from build123d import *


with BuildPart() as part:
    # Sweep1: sweep along a path in Sketch4
    with BuildLine(Plane(origin=(0, 0, 0), x_dir=(0, 0, -1), z_dir=(1, 0, 0))) as sweep1_path:
        Line((0, 0), (-2.286, 6.35))
    # Sketch2 → Sweep1 (sweep)
    with BuildSketch(Plane(origin=(0, 0, 0), x_dir=(1, 0, 0), z_dir=(0, 1, 0))):
        with BuildLine():
            Line((6.9596, -10.377746103), (4.0132, -10.377746103))
            Line((4.0132, -10.377746103), (4.0132, -5.373946103))
            Line((4.0132, -5.373946103), (2.413, -5.373946103))
            Line((2.413, -5.373946103), (3.556, -3.773746103))
            Line((3.556, -3.773746103), (-3.556, -3.773746103))
            Line((-3.556, -3.773746103), (-2.413, -5.373946103))
            Line((-2.413, -5.373946103), (-4.0132, -5.373946103))
            Line((-4.0132, -5.373946103), (-4.0132, -10.377746103))
            Line((-4.0132, -10.377746103), (-6.9596, -10.377746103))
            ThreePointArc((-6.9596, -10.377746103), (-5.806615649, -2.567356115), (-5.877729648, 5.327357779))
            ThreePointArc((-5.877729648, 5.327357779), (-5.125150102, 6.465638091), (-3.98686979, 5.713058545))
            ThreePointArc((-3.98686979, 5.713058545), (-2.834757288, 3.806705335), (-0.7366, 3.058853897))
            Line((-0.7366, 3.058853897), (-0.7366, 1.407853897))
            Line((-0.7366, 1.407853897), (0.7366, 1.407853897))
            Line((0.7366, 1.407853897), (0.7366, 3.058853897))
            ThreePointArc((0.7366, 3.058853897), (2.834757288, 3.806705335), (3.98686979, 5.713058545))
            ThreePointArc((3.98686979, 5.713058545), (5.125150102, 6.465638091), (5.877729648, 5.327357779))
            ThreePointArc((5.877729648, 5.327357779), (5.806615649, -2.567356115), (6.9596, -10.377746103))
        make_face()
    sweep(path=sweep1_path.line)


solid = part.part
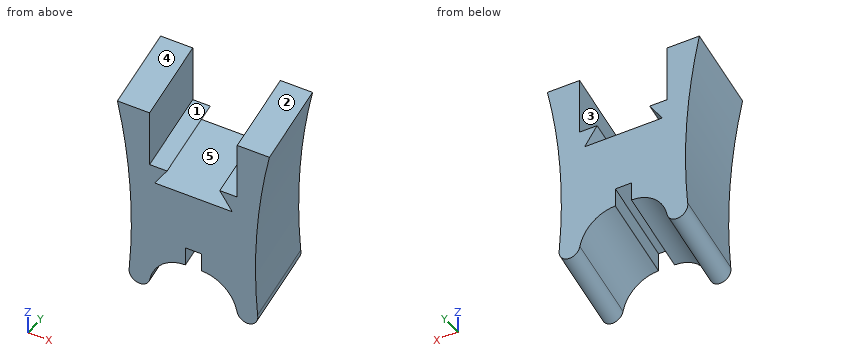
Read the model definition and answer for the solid it produces. Units are mm, in the model's axes. Face numbers are marked on the shaded views. A direction names the side the tool comes from. Round coordinates to 2 decimals unless told otherwise and drop trailing zeros. Write each loop counter-clockwise with the first axis right and the second up, starting at its lowest first coordinate (ties: lowest second). Pieces come first, ordered by that corner, then holes.
1. The part is cut by section A-A, the plane x = -0.5. Determine the outline of the cut face in (y, z), then the cut area to 3 significant figures.
2. Straight lines are drawn through the part: L1, parallel to X at y = 1.25, z = -3; L2, parallel to Z at x = -3, y = 2.5; L3, parallel to X at y = 1, z = -4.25. For each, find the intervals that lie inside material, in ascending order.
3. Given pin 1 Ø1.2 at (y, z) = (4.5, 0) entering from -X; pin 2 Ø4 at (x, z) = (-2.5, 8) entering from +Y; pin 3 Ø1.2 at (y, z) = (2.5, -0.5) entering from +X; pin 4 Ø3 at (x, y) = (5, 2.5) entering from -Z, each flat-ended and moving along its own axis, determine where each tip first touches the part or whether it passes through.
4. Determine the mould class of the marked faces 3, 4 and 5 for opening direction Z: pulls with the +Z half, pulls with the -Z half, needs draft (parallel to the pull), parting line crosses it, or undercut.
5. Which of the six approach directions +Z, -Z, +X, -X, +Y, -Y give full straight-line access (tool end or side, diameter ignored) to the marked faces 1 and 2?
Values:
1. outline: (0, -1.41) - (6.35, 0.88) - (6.35, 6.06) - (0, 3.77) - close
1. area: 32.9 mm2
2. L1: x = -5.75 to -2.3, 2.3 to 5.75
2. L2: z = -3.05 to 4.67, 5.45 to 6.27
2. L3: x = -5.82 to -3.54, 3.54 to 5.82
3. pin 1: stops at x = -5.7
3. pin 2: stops at y = 6.35
3. pin 3: stops at x = 5.7
3. pin 4: stops at z = -6.12
4. face 3: needs draft
4. face 4: pulls with the +Z half
4. face 5: undercut
5. face 1: +Z, -Y
5. face 2: +Z, +X, -X, -Y
